Could you check a few things on this drawing? It's one solid part, dimensions in mm from its lowest x, y, z. A direction names the side the tool comes from. Give positions to 0.01 mm unless a question says otherwise; leave off trailing zeros. Order: outer loops, then holes, each group sorted by start corner. A loop starts at its lowest first (then second) coordinate and runs counter-clockwise, first axis right, second up. Notation, with made-up numbers: (37, 79.5) -> (42, 79.5) arc R28 cw to (42, 104.5) -> close; hole circle Ø2 at (84, -36). An arc over 180 degrees is marked (long way). Answer as CSV lines item,"result".
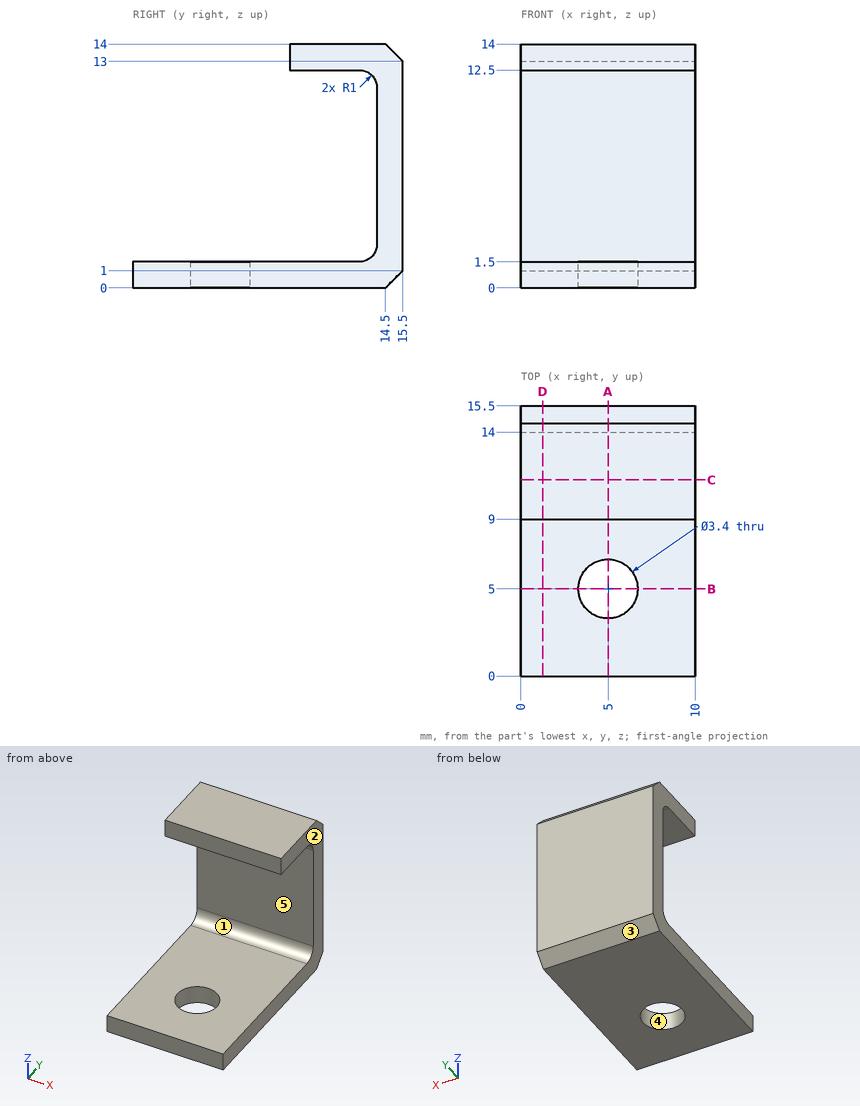
Item 1: We'd pull the mould along Z, two halves only. Please class the marked faces 3, 4 and 5: released by +Z, released by -Z, zero draft, split by the parting line, or undercut.
Numbers:
face 3,"released by -Z"
face 4,"zero draft"
face 5,"undercut"
Item 2: Imagine slicing it at B-B, the plane y = 5. Please give me the cut outline in (x, z).
Numbers:
outline,"(0, 0) -> (3.3, 0) -> (3.3, 1.5) -> (0, 1.5) -> close; (6.7, 0) -> (10, 0) -> (10, 1.5) -> (6.7, 1.5) -> close"
Item 3: Please list where these lines run through material, in increasing order: line 1 along Z through (x, y) = (6.25, 13); line 2 along Y through (x, z) = (5, 1.1); line 3 along Y through (x, z) = (0.5, 4.5).
Numbers:
line 1,"z = 0 to 1.5, 12.5 to 14"
line 2,"y = 0 to 3.3, 6.7 to 15.5"
line 3,"y = 14 to 15.5"
Item 4: For pin 1 (6 mm diameter, centred on x = 2, z = 7, fed in from -Y); pin 2 (1.2 mm diameter, centred on x = 3, z = 13.5, fed in from -Y); pin 3 (1.5 mm diameter, centred on x = 2.5, y = 8, fed in from +Z), each with a flat end and sliding along its axis, tell me the tip position at first contact or that it passes through.
Numbers:
pin 1,"stops at y = 14"
pin 2,"stops at y = 9"
pin 3,"stops at z = 1.5"
Item 5: Imagine slicing it at A-A, the plane x = 5. Please give me the cut outline in (y, z), then the cut area to 3 significant figures.
Numbers:
outline,"(0, 0) -> (3.3, 0) -> (3.3, 1.5) -> (0, 1.5) -> close; (6.7, 0) -> (14.5, 0) -> (15.5, 1) -> (15.5, 13) -> (14.5, 14) -> (9, 14) -> (9, 12.5) -> (13, 12.5) arc R1 cw to (14, 11.5) -> (14, 2.5) arc R1 cw to (13, 1.5) -> (6.7, 1.5) -> close"
area,"43.8 mm²"
Item 6: Imagine slicing it at C-C, the plane y = 11.25. Please give me the cut outline in (x, z).
Numbers:
outline,"(0, 0) -> (10, 0) -> (10, 1.5) -> (0, 1.5) -> close; (0, 12.5) -> (10, 12.5) -> (10, 14) -> (0, 14) -> close"
Item 7: For the marked faces 1 and 2, which set-ups out of +Z, -Z, +X, -X, +Y, -Y let a thin tool reach every point of the face, with its end or its side?
Numbers:
face 1,"+X, -X, -Y"
face 2,"+Z, -Z, +X, +Y, -Y"
Item 8: Imagine slicing it at D-D, the plane x = 1.25. Please give me the cut outline in (y, z).
Numbers:
outline,"(0, 0) -> (14.5, 0) -> (15.5, 1) -> (15.5, 13) -> (14.5, 14) -> (9, 14) -> (9, 12.5) -> (13, 12.5) arc R1 cw to (14, 11.5) -> (14, 2.5) arc R1 cw to (13, 1.5) -> (0, 1.5) -> close"
